Autodesk Inventor part; units mm, degrees
ref_plane "YZ Plane" through (0, 0, 0) normal (1, 0, 0) x (0, 1, 0)
ref_plane "XY Plane" through (0, 0, 0) normal (0, 0, 1) x (1, 0, 0)
sketch "Sketch1" plane through (0, 0, 0) normal (0, 1, 0) x (-1, 0, 0)
  arc A0 (0, -5) -> (0, 5) centre (0, 0) ccw
  line L0 (0, 5) -> (0, -5)
  dimension "d0" = 10
extrude "Extrusion1" add sketch "Sketch1" along normal blind 10
sketch "Sketch2" plane through (0, 0, 0) normal (1, 0, 0) x (0, 1, 0)
  line L0 (8.0172, -4.5) -> (8.0172, 4.5)
  line L1 (8.0172, 4.5) -> (2.5172, 4.5)
  line L2 (2.5172, -4.5) -> (0.0172, -2)
  line L3 (2.5172, 4.5) -> (0.0172, 2)
  line L4 (0.0172, -2) -> (0.0172, 2)
  line L5 (8.0172, -4.5) -> (2.5172, -4.5)
  point P0 (0, 0)
  dimension "d3" = 9
  dimension "d4" = 8
sketch "Sketch3" plane through (0, 0, 0) normal (1, 0, 0) x (0, 1, 0)
  line L0 (0, 2) -> (3, 5)
  arc A0 (3, 5) -> (0, 2) centre (1, 4) ccw
  line L1 (0, -2) -> (4, -6)
  arc A1 (0, -2) -> (4, -6) centre (1.75, -4.25) ccw
  line L2 (8.0325, 5) -> (11, 5)
  line L3 (11, 5) -> (11, -6)
  line L4 (11, -6) -> (8.0325, -6)
  line L5 (8.0325, -6) -> (8.0325, 5)
  line L6 (2.4911, 4.4911) -> (5, 7)
  line L7 (2.4911, 4.4911) -> (8.0325, 4.4911)
  arc A2 (8.0325, 4.4911) -> (5, 7) centre (7, 6.3303) ccw
  line L8 (2.4911, -4.4911) -> (8.5706, -4.4911)
  arc A3 (2.4911, -4.4911) -> (8.5706, -4.4911) centre (5.5309, -7.5041) ccw
  point P0 (0, 0)
extrude "Extrusion2" cut sketch "Sketch3" against normal through all
sketch "Sketch4" plane through (0, 0, 0) normal (0, 1, 0) x (-1, 0, 0)
  arc A0 (1.0726, -4.4911) -> (1.0726, 4.4911) centre (-1.125, 0) ccw
  arc A1 (1.0726, 4.4911) -> (1.0726, -4.4911) centre (-0.4517, 0) ccw
  point P0 (0, 0)
  point P1 (2.1976, -4.4911)
  point P2 (2.1976, 4.4911)
  dimension "d9" = 1.125
  dimension "d10" = 1.125
extrude "Extrusion3" cut sketch "Sketch4" along normal through all both and the other way through all
sketch "Sketch5" plane through (0, 0, 0) normal (1, 0, 0) x (0, 1, 0)
  line L0 (1.6, -1.2445) -> (1.6, 1.1555)
  line L1 (6.4325, 2.6911) -> (3.1125, 2.6911)
  line L2 (6.4325, -2.6911) -> (6.4325, 2.6911)
  line L3 (6.4325, -2.6911) -> (3.1125, -2.6911)
  line L4 (0, 2) -> (0, -2)
  line L5 (8.0325, 4.4911) -> (8.0325, -4.4911)
  line L6 (0, 2) -> (2.4911, 4.4911)
  line L7 (2.4911, 4.4911) -> (8.0325, 4.4911)
  line L8 (8.0325, 4.4911) -> (8.0325, -4.4911)
  line L9 (8.0325, -4.4911) -> (2.4911, -4.4911)
  line L10 (2.4911, -4.4911) -> (0, -2)
  line L11 (0, 2) -> (0, -2)
  line L12 (1.6, 1.1555) -> (3.1125, 2.6911)
  line L13 (1.6, -1.2445) -> (3.1125, -2.6911)
  line L14 (1.6, 4.6579) -> (1.6, -5.3823)
  arc A0 (1.6, 4.6579) -> (1.6, -5.3823) centre (3.2437, -0.3622) ccw
  line L15 (1.6, 1.1555) -> (5.4757, 5.0906)
  line L16 (1.6, 1.1555) -> (1.6, 7.5999)
  arc A1 (5.4757, 5.0906) -> (1.6, 7.5999) centre (3.8837, 6.8794) ccw
  line L17 (3.1125, 2.6911) -> (12.4034, 2.6911)
  line L18 (3.1125, 2.6911) -> (8.5318, 8.1936)
  arc A2 (12.4034, 2.6911) -> (8.5318, 8.1936) centre (8.3272, 3.9364) ccw
  line L19 (6.4325, 2.6911) -> (13.6333, 2.6911)
  line L20 (6.4325, 2.6911) -> (6.4325, -9.3636)
  arc A3 (6.4325, -9.3636) -> (13.6333, 2.6911) centre (6.37, -1.1482) ccw
  line L21 (6.4325, -2.6911) -> (6.4325, -11.5775)
  line L22 (6.4325, -2.6911) -> (3.1125, -2.6911)
  line L23 (3.1125, -2.6911) -> (3.2437, -12.8567)
  arc A4 (3.2437, -12.8567) -> (6.4325, -9.3636) centre (5.6123, -11.8169) ccw
  line L24 (1.6, -1.2445) -> (1.6, -8.2222)
  line L25 (1.6, -1.2445) -> (3.1125, -2.6911)
  line L26 (3.1125, -2.6911) -> (3.1946, -9.0574)
  arc A5 (1.6, -8.2222) -> (3.1946, -9.0574) centre (2.6381, -8.1801) ccw
  point P0 (0, 0)
  dimension "d16" = 1.6
  dimension "d18" = 1.6
  dimension "d21" = 1.8
  dimension "d23" = 1.8
  dimension "d24" = 2.4
  dimension "d26" = 3.32
  dimension "d27" = 3.32
extrude "Extrusion4" cut sketch "Sketch5" against normal through all contours L14 L10 L4 L6 L0 | L13 L23 L9 L10 L14 | L14 L6 L7 L15 L12 | L3 L20 L9 L23 | L14 A0 L6 L4 L10 | L10 L9 L23 A5 L24 L14 | L15 L7 L5 L17 L1 | L14 L16 A1 L15 L7 L6 | L2 L17 L5 L9 L20 | L9 L20 A4 L23 | L15 L18 A2 L17 L5 L7 | L9 L5 L17 L19 A3 L20
sketch "Sketch6" plane through (0, 0, 0) normal (1, 0, 0) x (0, 1, 0)
  circle A0 centre (4, 0) radius 2.5
  line L0 (1.6, -1.2445) -> (1.6, 1.1555)
  point P0 (0, 0)
  dimension "d31" = 5
  dimension "d32" = 2.4
extrude "Extrusion5" add sketch "Sketch6" against normal blind 15
sketch "Sketch7" plane through (0, 0, 0) normal (0, 1, 0) x (-1, 0, 0)
  arc A0 (3.089, -2.6911) -> (3.7176, -1.2445) centre (-1.125, 0) ccw
  arc A1 (3.7397, 1.1555) -> (3.089, 2.6911) centre (-1.125, 0) ccw
  arc A2 (3.7176, -1.2445) -> (3.7397, 1.1555) centre (-1.125, 0) ccw
  arc A3 (3.089, 2.6911) -> (3.089, -2.6911) centre (1.3425, 0) ccw
  point P0 (0, 0)
extrude "Extrusion6" cut sketch "Sketch7" along normal through all
sketch "Sketch8" plane through (-15, 4, 0) normal (-1, 0, 0) x (0, 0, 1)
  circle A0 centre (0, 0) radius 0.5875
  point P0 (0, -4)
  dimension "d37" = 1.175
extrude "Extrusion7" cut sketch "Sketch8" against normal blind 7
sketch "Sketch9" plane through (0, 0, 0) normal (0, 1, 0) x (-1, 0, 0)
  line L0 (6, 3) -> (2, 3)
  line L1 (2, 3) -> (2, -3)
  line L2 (2, -3) -> (6, -3)
  line L3 (6, -3) -> (6, 3)
  point P0 (0, 0)
extrude "Extrusion8" cut sketch "Sketch9" along normal through all both and the other way through all
sketch "Sketch10" plane through (-15, 4, 0) normal (-1, 0, 0) x (0, 0, 1)
  circle A0 centre (0, 0) radius 1.25
  circle A1 centre (0, 0) radius 3.9528
  point P0 (0, -4)
  dimension "d67" = 2.5
extrude "Extrusion9" cut sketch "Sketch10" against normal blind 8
ref_plane "Work Plane1" through (0, 4.1, 0) normal (0, 1, 0) x (-1, 0, 0)
sketch "Sketch12" plane through (0, 4.1, 0) normal (0, 1, 0) x (-1, 0, 0)
  line L0 (15, -1) -> (15, 1)
  line L1 (5.9669, 12.7) -> (5.9669, -12.7)
  line L2 (5.9669, 12.7) -> (-93.99, 0)
  line L3 (-93.99, 0) -> (5.9669, -12.7)
  line L4 (7.0341, 14.6962) -> (7.0341, -14.7038)
  line L5 (2.03, -0.0038) -> (19.03, -0.0038)
  line L6 (-97, 5.0008) -> (-97, -4.9992)
  line L7 (7.0341, 14.6962) -> (-97, 5.0008)
  line L8 (7.0341, -14.7038) -> (-97, -4.9992)
  point P0 (0, 0)
  point P1 (0, 0)
  dimension "d61" = 25.4
  dimension "d62" = 29.4
  dimension "d63" = 14.7
  dimension "d64" = 10
extrude "Extrusion11" add sketch "Sketch12" along normal mid plane 1.5
properties part number "piezo_mounted_whisk_deflector_LONG"
The listing builds one solid part. Answer for the finished solid, in the listing's coordinates (mm). A direction names the side the tool comes from. Coordinates: 2 decimals unless noted, no trailing zeros. Write each loop counter-clockwise with the first axis right and the second up, starting at its lowest first coordinate (ties: lowest second). Pieces come first, ordered by that corner, then holes. Notation, with made-up numbers: (-4, 55.5) - (47, 55.5) arc R30 cw to (47, 94.5) - close; hole circle Ø11 at (20.25, 76). An arc over 180 degrees is marked (long way). Put each result on its own line as item: value.
1. Determine the mould class of faces 3 (the face through (-7, 2, 0)), 4 (the face through (44.71, 4.09, -6.26)), 5 (the face through (43.31, 4.09, 6.44)), 6 (the face through (52.9, 4.85, -5.4)) for opening direction X: pulls with the +X half, pulls with the -X half, needs draft (parallel to the pull), parting line crosses it, or undercut.
Answer sheet:
face 3: pulls with the -X half
face 4: undercut
face 5: undercut
face 6: needs draft
2. A tool of negligible diameter and unlimited length cuts with its end or side. For faces 1 (the face through (-15, 4, -1)), 2 (the face through (-11.06, 2.78, -0.27)), from which of +Z, -Z, +X, -X, +Y, -Y can it reach the whole face along a straight path? Write none if from no direction.
Answer sheet:
face 1: +Z, -Z, -X, +Y, -Y
face 2: -X
3. Find the intervals of material crossed by line 1 along Y through (x, z) = (-11.5, 0); line 2 along Y through (x, z) = (21, 11.25); line 3 along Z through (x, y) = (39.5, 4.7), in increasing order. Write a range as from..to.
Answer sheet:
line 1: y = 2.75..3.41, 4.59..5.25
line 2: y = 3.35..4.85
line 3: z = -10.36..-6.92, 6.92..10.36
4. The part is cut by section A-A on x = 87.5. Give the vertices of the cut face in (y, z).
Answer sheet:
outline: (3.35, -5.89) - (4.85, -5.89) - (4.85, -0.82) - (3.35, -0.82) - close; (3.35, 0.82) - (4.85, 0.82) - (4.85, 5.89) - (3.35, 5.89) - close
5. Flat-ended cylindrical pins translate along their axes: pin 1 Ø0.6 at (y, z) = (4, 0) entering from -X; pin 2 Ø2 at (x, z) = (60, 6) entering from -Y; pin 3 Ø2 at (y, z) = (2, 2.5) entering from +X; pin 4 Ø2 at (y, z) = (6, 0) entering from -X. Find the tip coordinate at first contact, or state that the pin passes through.
Answer sheet:
pin 1: stops at x = -8
pin 2: stops at y = 3.35
pin 3: stops at x = -6
pin 4: stops at x = -15
6. The part is cut by section B-B on z = -11. Give the vertices of the cut face in (x, y).
Answer sheet:
outline: (-7.03, 3.35) - (-5.97, 3.35) - (-5.97, 4.85) - (-7.03, 4.85) - close; (7.41, 3.35) - (32.67, 3.35) - (32.67, 4.85) - (7.41, 4.85) - close
